Source: CAD feature listing. Evaluate the final solid. Frame: model axes, mm. A direction names the side the tool comes from. Coordinates: 2 decimals unless noted, no trailing zeros. Order: outer loops, then holes, each group sorted by start corner. A loop starts at its lowest first (then second) coordinate and runs counter-clockwise, first axis right, second up.
```python
from build123d import *

# Parameters (mm, degrees)
SKETCH2_R           = 12.7
BOSS_EXTRUDE1_DEPTH = 12


with BuildPart() as part:
    # Sketch1 → Revolve1 (revolve)
    with BuildSketch(Plane(origin=(0, 0, 0), x_dir=(1, 0, 0), z_dir=(0, 1, 0))):
        with BuildLine():
            Line((12.7, 0), (25.4, 0))
            Line((25.4, 0), (25.4, 2.825))
            ThreePointArc((25.4, 2.825), (22.225, 6), (25.4, 9.175))
            Line((25.4, 9.175), (25.4, 12))
            Line((25.4, 12), (12.7, 12))
            Line((12.7, 12), (12.7, 0))
        make_face()
    revolve(axis=Axis((0, 0, 0), (0, 0, -1)))

    # Sketch2 → Boss-Extrude1 (add)
    with BuildSketch(Plane.XY):
        Circle(SKETCH2_R)
        Polygon((3.609388519, -5.225480634), (6.330093235, 0.513081832), (2.720704717, 5.738562466), (-3.609388519, 5.225480634), (-6.330093235, -0.513081832), (-2.720704717, -5.738562466), align=None, mode=Mode.SUBTRACT)
    extrude(amount=-BOSS_EXTRUDE1_DEPTH)


solid = part.part
```
Q1. Pull-direction query (X, two-part tool) for faces 3 (the flat face through (0, 6, -12)), 4 (the cylindrical face through (-5.506, 24.796, -10.607)), 5 (the flat face through (4.95, -2.4, -5.92)); classes: pulls with the +X half, pulls with the -X half, needs draft (parallel to the pull), parting line crosses it, or undercut.
Solutions:
face 3: needs draft
face 4: parting line crosses it
face 5: undercut
Q2. Section query A-A on z = -1.5. Output: boundary loops of the cut face in (x, y).
Solutions:
outline: circle Ø50.8 at (0, 0); hole (-6.33, -0.51) - (-2.72, -5.74) - (3.61, -5.23) - (6.33, 0.51) - (2.72, 5.74) - (-3.61, 5.23) - close
Q3. Section query B-B on x = 0. Output: boundary loops of the cut face in (y, z) (3 decimals).
Solutions:
outline: (-25.4, -12) - (-5.518, -12) - (-5.518, 0) - (-25.4, 0) - (-25.4, -2.825) arc R3.175 cw to (-25.4, -9.175) - close; (5.518, -12) - (25.4, -12) - (25.4, -9.175) arc R3.175 cw to (25.4, -2.825) - (25.4, 0) - (5.518, 0) - close
Q4. Section query C-C on z = -4.5. Output: boundary loops of the cut face in (x, y).
Solutions:
outline: circle Ø45.2 at (0, 0); hole (-6.33, -0.51) - (-2.72, -5.74) - (3.61, -5.23) - (6.33, 0.51) - (2.72, 5.74) - (-3.61, 5.23) - close
Q5. Material intervals for line 1 along X through (y, z) = (-2.5, -4); line 2 along X through (y, z) = (5, -9.75); line 3 along Y through (x, z) = (3.5, -10), sorted ascending.
Solutions:
line 1: x = -22.8 to -4.96, 4.9 to 22.8
line 2: x = -24.9 to -3.72, 3.23 to 24.9
line 3: y = -25.16 to -5.23, 4.61 to 25.16
Q6. Pin query (flat end, axial travel): P1, Ø1, axis at y = 8, z = -10.5, coming from the -X side; P2, Ø4, axis at x = 19.5, z = -1.5, coming from the -Y side; P3, Ø1.5, axis at y = 2, z = -7.5, coming from the +X side. Return the tip coordinate at first contact, or that it passes through.
Solutions:
P1: stops at x = -24.27
P2: stops at y = -18.41
P3: stops at x = 23.08
Q7. Set-up query: faces 1 (the flat face through (0, 6, 0)), 2 (the flat face through (-4.55, -3.09, -5.92)). Return all of +Z, -Z, +X, -X, +Y, -Y with unobstructed straight access to the full face (end or side cutting, diameter ignored); none if empty.
Solutions:
face 1: +Z, +X, -X, +Y, -Y
face 2: +Z, -Z
